```python
from build123d import *

# Parameters (mm, degrees)
F2_W     = 34
F2_H     = 23.5
F4_W     = 10
F4_H     = 12
F5_DEPTH = 200.001
F6_W     = 2.15
F6_H     = 10
F6_W_2   = 2.65


with BuildPart() as f1:
    # F0 (on Front) → F1 (revolve)
    with BuildSketch(Plane.XZ):
        Polygon((0, 27.5), (0, 20), (200, 20), (200, 27.5), (172, 27.5), (172, 36), (74.5, 36), (74.5, 40), (62.5, 40), (62.5, 35), (27.5, 35), (27.5, 27.5), align=None)
    revolve(axis=Axis((44.474047, 0, 0), (1, 0, 0)))

    # F2 (on Front) → F3 (revolve, cut)
    with BuildSketch(Plane.XZ):
        with Locations((100, 11.75)):
            Rectangle(F2_W, F2_H)
    revolve(axis=Axis((100, 0, 0), (1, 0, 0)), mode=Mode.SUBTRACT)

    # F4 (on face) → F5 (cut, through all)
    with BuildSketch(Plane.YZ.offset(200)):
        with Locations((17.4, 0)):
            Rectangle(F4_W, F4_H)
    extrude(amount=-F5_DEPTH, mode=Mode.SUBTRACT)

    # F6 (on Front) → F7 (revolve, cut)
    with BuildSketch(Plane.XZ):
        with Locations((8.425, 31)):
            Rectangle(F6_W, F6_H)
        with Locations((191.075, 31)):
            Rectangle(F6_W, F6_H)
        with Locations((146.175, 39.5)):
            Rectangle(F6_W_2, F6_H)
    revolve(axis=Axis((18.830039, 0, 0), (1, 0, 0)), mode=Mode.SUBTRACT)


solid = f1.part
```
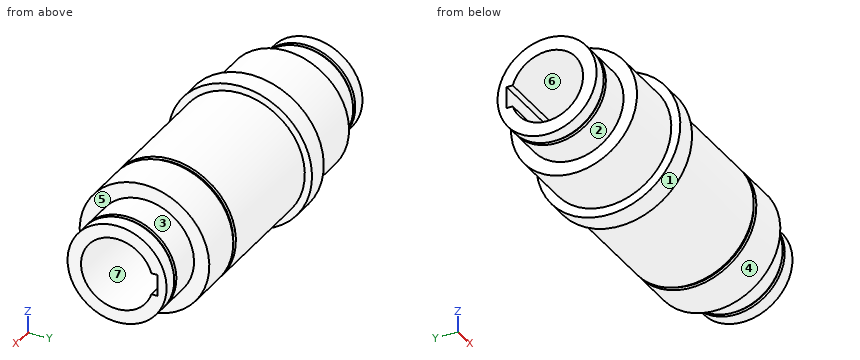
The model under review builds one solid part; all positions refer to its coordinate system, in mm. Face numbers are marked on the shaded views. A direction names the side the tool comes from. Coordinates: 2 decimals unless noted, no trailing zeros. Write each loop counter-clockwise with the first axis right and the second up, starting at its lowest first coordinate (ties: lowest second). Pieces come first, ordered by that corner, then holes.
1) Machinability: for the marked faces 1, 2 and 3, which of the approach directions +Z, -Z, +X, -X, +Y, -Y give a long, thin tool a straight path to every point of the face, cutting with its end or side? Answer none if there is none.
2) The part is to be moulded in two halves that separate along Z. For the marked faces 4, 5, 6 and 7, say which applies: pulls with the +Z half, pulls with the -Z half, needs draft (parallel to the pull), parting line crosses it, or undercut.
3) Clearance check with flat-ended pins moving along their axes: pin 1 Ø9.5 at (x, z) = (35, 0) entering from -Y; pin 2 Ø21.5 at (y, z) = (-3, -2.5) entering from +X; pin 3 Ø1.7 at (x, y) = (29, 20.5) entering from -Z; pin 4 Ø3.5 at (x, z) = (150.5, 1.5) entering from -Y. State where each tip first meets the part, or that it passes through.
4) To check wall thickness, follow probe 1 along X at (y, z) = (7, -35); probe 2 along Z at (x, y) = (18, 0); probe 3 along Z at (x, y) = (30.5, 0). State the ranges of each line that lie inside material, in increasing order.
5) We need section B-B on z = -32. State the section outline as (x, y) points.
6) We need section A-A on x = 120. State the section outline as (y, z) points.
Answer list:
1. face 1: +X, -X
1. face 2: -X
1. face 3: +X
2. face 4: parting line crosses it
2. face 5: needs draft
2. face 6: undercut
2. face 7: undercut
3. pin 1: stops at y = -35
3. pin 2: passes through
3. pin 3: stops at z = -28.96
3. pin 4: stops at y = -36
4. probe 1: x = 62.5 to 144.85, 147.5 to 172
4. probe 2: z = -27.5 to -20, 20 to 27.5
4. probe 3: z = -35 to -20, 20 to 35
5. outline: (27.5, -14.18) - (62.5, -14.18) - (62.5, -24) - (74.5, -24) - (74.5, -16.49) - (144.85, -16.49) - (144.85, -12.89) - (147.5, -12.89) - (147.5, -16.49) - (172, -16.49) - (172, 16.49) - (147.5, 16.49) - (147.5, 12.89) - (144.85, 12.89) - (144.85, 16.49) - (74.5, 16.49) - (74.5, 24) - (62.5, 24) - (62.5, 14.18) - (27.5, 14.18) - close
6. outline: circle Ø72 at (0, 0); hole (19.08, -6) - (22.4, -6) - (22.4, 6) - (19.08, 6) arc R20 ccw (long way) to start
